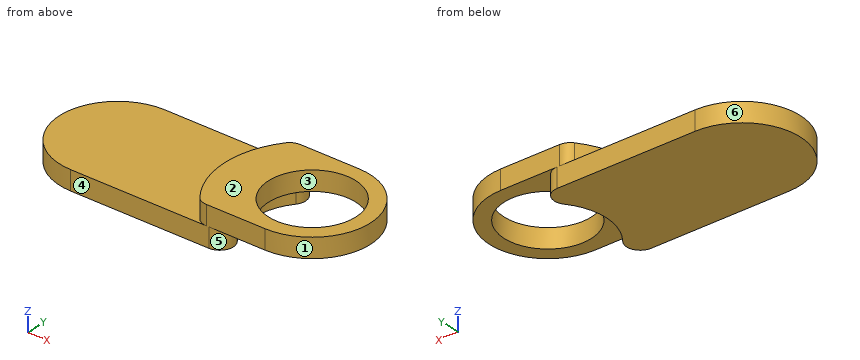
from build123d import *

# Parameters (mm, degrees)
SKETCH_1_R           = 3
SKETCH_1_R_2         = 2.25
EXTRUDE_1_DEPTH      = 1
EXTRUDE_2_DEPTH      = 1
EXTRUDE_2_DEPTH_BACK = 1
CUT_EXTRUDE_1_DEPTH  = 1
FILLET_START         = -2
FILLET_1_DEPTH       = 2
FILLET_2_R           = 0.7


with BuildPart() as part:
    # 草图1 → 凸台-拉伸1 (new body)
    with BuildSketch(Plane.XY):
        Circle(SKETCH_1_R)
        Circle(SKETCH_1_R_2, mode=Mode.SUBTRACT)
    extrude(amount=EXTRUDE_1_DEPTH)

    # 草图2 → 凸台-拉伸2 (add, two sides: drawn at the far end of the back side and taken through both)
    with BuildSketch(Plane(origin=(0, 0, 0), x_dir=(-1, 0, 0), z_dir=(0, 0, -1)).offset(-EXTRUDE_2_DEPTH_BACK)):
        with BuildLine():
            Line((0, -3), (10, -3))
            ThreePointArc((10, -3), (13, 0), (10, 3))
            Line((10, 3), (0, 3))
            ThreePointArc((0, 3), (3, 0), (0, -3))
        make_face()
    extrude(amount=EXTRUDE_2_DEPTH + EXTRUDE_2_DEPTH_BACK)

    # 草图3 → 切除-拉伸1 (cut)
    with BuildSketch(Plane(origin=(0, 0, 1), x_dir=(-1, 0, 0), z_dir=(0, 0, -1))):
        with BuildLine():
            Line((3.354101966, -3), (10, -3))
            ThreePointArc((10, -3), (13, 0), (10, 3))
            Line((10, 3), (3.354101966, 3))
            ThreePointArc((3.354101966, 3), (4.5, 0), (3.354101966, -3))
        make_face()
    extrude(amount=CUT_EXTRUDE_1_DEPTH, mode=Mode.SUBTRACT)

    # 圆角1: read off the stored shape, not the designer's step
    # 圆角1 outline → 圆角1 (cut)
    with BuildSketch(Plane.XY.offset(FILLET_START)):
        with BuildLine():
            ThreePointArc((0, -3), (-1.304876509, -2.701351013), (-2.349952986, -1.864864865))
            ThreePointArc((-2.349952986, -1.864864865), (-2.267960113, -2.604471185), (-2.898275349, -3))
            Line((-2.898275349, -3), (0, -3))
        make_face()
        with BuildLine():
            ThreePointArc((-2.898275349, 3), (-2.267960113, 2.604471185), (-2.349952986, 1.864864865))
            ThreePointArc((-2.349952986, 1.864864865), (-1.304876509, 2.701351013), (0, 3))
            Line((0, 3), (-2.898275349, 3))
        make_face()
    extrude(amount=FILLET_1_DEPTH, mode=Mode.SUBTRACT)

    # 圆角2
    fillet_2_edges = [part.edges().sort_by_distance(p)[0] for p in [
        (-3.354101966, 3, 0.5),
        (-3.354101966, -3, 0.5),
    ]]
    fillet(fillet_2_edges, radius=FILLET_2_R)


solid = part.part
Work out the finished part from the listing and answer in its coordinate system (mm). Face numbers are marked on the shaded views. A direction names the side the tool comes from. Coordinates: 2 decimals unless noted, no trailing zeros. Loops run counter-clockwise (first coordinate to the right, second up) from the corner with the lowest first, then second, coordinate; pieces in that order, holes last. Notation, with made-up numbers: (83, 83.5) -> (108, 83.5) arc R19 ccw to (108, 115.5) -> close; hole circle Ø5 at (30, 16). An arc over 180 degrees is marked (long way). Write each question's results on one line, items separated by ' | '. Start each with the question number.
1) A flat-ended cylindrical pin translates along its axis: P1, Ø1.8, axis at x = -9, y = -1, coming from the +Z side. Find the tip coordinate at first contact, or state that the pin passes through.
2) Find section D-D on x = -7.75. Determine the outline of the cut face in (y, z), then the cut area to 3 significant figures.
3) Find section C-C on y = -0.7. Determine the outline of the cut face in (x, z), then the cut area to 3 significant figures.
4) The mould has two halves that part along Y. Classify the marked faces 1, 2, 3 and 4: pulls with the +Y half, pulls with the -Y half, needs draft (parallel to the pull), parting line crosses it, or undercut.
5) Find section A-A on y = 0. Determine the outline of the cut face in (x, z), then the cut area to 3 significant figures.
6) Consider line 1 along Y through (x, z) = (0, 0.4); line 2 along Z through (x, y) = (-11.75, 1.7); line 3 along X through (y, z) = (-0.25, 0.85). Determine where each line is inside the solid, lowest interval first.
7) Find section B-B on z = 0.2. Determine the outline of the cut face in (x, y), then the cut area to 3 significant figures.
8) For the marked faces 5 and 6, determine the directions among +Z, -Z, +X, -X, +Y, -Y from which every point of the face is accessible in a straight line to the end or side of a thin tool.
Response values:
1) P1: stops at z = 0
2) outline: (-3, -1) -> (3, -1) -> (3, 0) -> (-3, 0) -> close | area: 6.00 mm^2
3) outline: (-12.92, -1) -> (-2.92, -1) -> (-2.92, 0) -> (-2.14, 0) -> (-2.14, 1) -> (-4.45, 1) -> (-4.45, 0) -> (-12.92, 0) -> close; (2.14, 0) -> (2.92, 0) -> (2.92, 1) -> (2.14, 1) -> close | area: 13.1 mm^2
4) face 1: parting line crosses it | face 2: needs draft | face 3: undercut | face 4: pulls with the -Y half
5) outline: (-13, -1) -> (-3, -1) -> (-3, 0) -> (-2.25, 0) -> (-2.25, 1) -> (-4.5, 1) -> (-4.5, 0) -> (-13, 0) -> close; (2.25, 0) -> (3, 0) -> (3, 1) -> (2.25, 1) -> close | area: 13.0 mm^2
6) line 1: y = -3 to -2.25, 2.25 to 3 | line 2: z = -1 to 0 | line 3: x = -4.49 to -2.24, 2.24 to 2.99
7) outline: (-3.58, -2.72) arc R0.7 ccw to (-3.02, -3) -> (0, -3) arc R3 ccw to (0, 3) -> (-3.02, 3) arc R0.7 ccw to (-3.58, 2.72) arc R4.5 ccw to start; hole circle Ø4.5 at (0, 0) | area: 23.0 mm^2
8) face 5: -Z, +X | face 6: +Z, -Z, -X
